from build123d import *

# Parameters (mm, degrees)
F1_DEPTH = 12.7
F2_SIZE  = 1.5875
F3_R     = 3.175
F8_ANGLE = 90


with BuildPart() as f1:
    # F0 (on Top) → F1 (new body)
    with BuildSketch(Plane.XY):
        with BuildLine():
            Line((25.4, 20.6375), (-12.7, 20.6375))
            ThreePointArc((-12.7, 20.6375), (-21.6802561211, 16.9177561211), (-25.4, 7.9375))
            Line((-25.4, 7.9375), (-25.4, -20.6375))
            Line((-25.4, -20.6375), (25.4, -20.6375))
            Line((25.4, -20.6375), (25.4, -5.55625))
            Line((25.4, -5.55625), (22.1241805311, -5.55625))
            ThreePointArc((22.1241805311, -5.55625), (21.2950640303, -7.0075640303), (19.84375, -7.8366805311))
            Line((19.84375, -7.8366805311), (19.84375, -11.2133194689))
            ThreePointArc((19.84375, -11.2133194689), (21.5600578928, -12.3432175167), (22.225, -14.2875))
            ThreePointArc((22.225, -14.2875), (17.1057175167, -16.7975578928), (18.25625, -11.2133194689))
            Line((18.25625, -11.2133194689), (18.25625, -7.8366805311))
            ThreePointArc((18.25625, -7.8366805311), (15.875, -4.7625), (18.25625, -1.6883194689))
            Line((18.25625, -1.6883194689), (18.25625, 1.6883194689))
            ThreePointArc((18.25625, 1.6883194689), (15.875, 4.7625), (18.25625, 7.8366805311))
            Line((18.25625, 7.8366805311), (18.25625, 11.2133194689))
            ThreePointArc((18.25625, 11.2133194689), (17.1057175167, 16.7975578928), (22.225, 14.2875))
            ThreePointArc((22.225, 14.2875), (21.5600578928, 12.3432175167), (19.84375, 11.2133194689))
            Line((19.84375, 11.2133194689), (19.84375, 7.8366805311))
            ThreePointArc((19.84375, 7.8366805311), (21.5600578928, 6.7067824833), (22.225, 4.7625))
            ThreePointArc((22.225, 4.7625), (21.5600578928, 2.8182175167), (19.84375, 1.6883194689))
            Line((19.84375, 1.6883194689), (19.84375, -1.6883194689))
            ThreePointArc((19.84375, -1.6883194689), (21.2950640303, -2.5174359697), (22.1241805311, -3.96875))
            Line((22.1241805311, -3.96875), (25.4, -3.96875))
            Line((25.4, -3.96875), (25.4, 20.6375))
        make_face()
        Polygon((-5.3676515813, 7.9375), (-9.0338257906, 1.5875), (-16.3661742094, 1.5875), (-20.0323484187, 7.9375), (-16.3661742094, 14.2875), (-9.0338257906, 14.2875), align=None, mode=Mode.SUBTRACT)
        with BuildLine():
            Line((19.84375, -11.2133194689), (19.84375, -7.8366805311))
            ThreePointArc((19.84375, -7.8366805311), (19.05, -7.9375), (18.25625, -7.8366805311))
            Line((18.25625, -7.8366805311), (18.25625, -11.2133194689))
            ThreePointArc((18.25625, -11.2133194689), (19.05, -11.1125), (19.84375, -11.2133194689))
        make_face()
        with BuildLine():
            ThreePointArc((18.25625, -1.6883194689), (19.05, -1.5875), (19.84375, -1.6883194689))
            Line((19.84375, -1.6883194689), (19.84375, 1.6883194689))
            ThreePointArc((19.84375, 1.6883194689), (19.05, 1.5875), (18.25625, 1.6883194689))
            Line((18.25625, 1.6883194689), (18.25625, -1.6883194689))
        make_face()
    extrude(amount=F1_DEPTH)

    # F2
    f2_edges = [f1.edges().sort_by_distance(p)[0] for p in [
        (19.05, 1.5875, 12.7),
        (19.05, 17.4625, 12.7),
        (18.25625, 9.525, 12.7),
        (19.84375, 9.525, 12.7),
    ]]
    chamfer(f2_edges, length=F2_SIZE)

    # F3
    f3_edges = [f1.edges().sort_by_distance(p)[0] for p in [
        (-7.200739, 4.7625, 12.7),
        (-7.200739, 11.1125, 12.7),
        (-12.7, 14.2875, 12.7),
        (-18.199261, 11.1125, 12.7),
        (-18.199261, 4.7625, 12.7),
        (-12.7, 1.5875, 12.7),
        (-16.366174, 14.2875, 6.35),
        (-20.032348, 7.9375, 6.35),
        (-16.366174, 1.5875, 6.35),
        (-9.033826, 1.5875, 6.35),
        (-5.367652, 7.9375, 6.35),
        (-9.033826, 14.2875, 6.35),
    ]]
    fillet(f3_edges, radius=F3_R)

    # F5 (on face) → F6 section 0
    with BuildSketch(Plane(origin=(0, 0, 0), x_dir=(1, 0, 0), z_dir=(0, 0, -1))):
        Polygon((-6.35, 11.0185455743), (-6.35, 3.6861971556), (0, 0.0200229463), (6.35, 3.6861971556), (6.35, 11.0185455743), (0, 14.6847197837), align=None)
    # F4 (on face) → F6 section 1
    with BuildSketch(Plane.XY.offset(12.7)):
        Polygon((2.749630657, -2.589871365), (-2.749630657, -2.589871365), (-5.499261314, -7.352371365), (-2.749630657, -12.114871365), (2.749630657, -12.114871365), (5.499261314, -7.352371365), align=None)
    loft(mode=Mode.SUBTRACT)

    # F7 (on face) → F8 (revolve)
    with BuildSketch(Plane.XZ.offset(20.6375)):
        with BuildLine():
            Line((-25.4, 12.7), (-6.35, 12.7))
            ThreePointArc((-6.35, 12.7), (-15.875, 22.225), (-25.4, 12.7))
        make_face()
    revolve(axis=Axis((-15.875, -20.6375, 12.7), (-1, 0, 0)), revolution_arc=F8_ANGLE)


solid = f1.part
Can you work these out from the model? Positions are in its coordinate system, mm. A direction names the side the tool comes from. Give positions to 0.01 mm unless a question says otherwise; leave off trailing zeros. Loops run counter-clockwise (first coordinate to the right, second up) from the corner with the lowest first, then second, coordinate; pieces in that order, holes last. Notation, with made-up numbers: (59, -31.75) - (81, -31.75) arc R32 cw to (81, 5.25) - close; hole circle Ø7 at (58, 32). An arc over 180 degrees is marked (long way). Return JSON: item names as keys, results as strings.
1. I'm going to push flat-ended pins straight in: pin 1 Ø1.7 at (y, z) = (10, 5) entering from -X; pin 2 Ø2 at (x, y) = (-19.5, -16) entering from +Z; pin 3 Ø20.5 at (x, y) = (1, -5) entering from +Z. Where does each tip first touch, or does it pass through?
Output values:
{"pin 1": "stops at x = -25.34", "pin 2": "stops at z = 20.88", "pin 3": "stops at z = 12.7"}
2. I want a section at A-A on x = 19.05. Please give me the cut outline in (y, z), and give its area (3 significant figures).
Output values:
{"outline": "(-20.64, 0) - (-17.46, 0) - (-17.46, 12.7) - (-20.64, 12.7) - close; (-11.11, 0) - (-7.94, 0) - (-7.94, 12.7) - (-11.11, 12.7) - close; (-1.59, 0) - (1.59, 0) - (1.59, 11.11) - (0, 12.7) - (-1.59, 12.7) - close; (17.46, 0) - (20.64, 0) - (20.64, 12.7) - (19.05, 12.7) - (17.46, 11.11) - close", "area": "159 mm²"}
3. We'd pull the mould along Y, two halves only. Please class faces 1 (the face through (-6, -20.638, 9)), 2 (the face through (-5.86, 7.96, 4.83)), 3 (the face through (25.4, -13, 6)): +Y half, -Y half, draft (parallel to the pull), parting line (faces both ways), or undercut.
Output values:
{"face 1": "-Y half", "face 2": "undercut", "face 3": "draft"}
4. If I drill on line 1 (Y direction, x = 19.05, z = 8.25); line 2 (Y direction, x = -12, z = 6.5); line 3 (Z direction, x = 17, y = 0), over which ranges is the centre line in solid material (lowest first)?
Output values:
{"line 1": "y = -20.64 to -17.46, -11.11 to -7.94, -1.59 to 1.59, 17.46 to 20.64", "line 2": "y = -20.64 to 1.59, 14.29 to 20.64", "line 3": "z = 0 to 12.7"}
5. I want a section at C-C on z = 1.5. Give the number of separate pieces and of enclosed holes in the cut face, and give its area (3 significant figures).
Output values:
{"separate pieces": "1", "enclosed holes": "4", "area": "1,660 mm²"}
6. For faces 4 (the face through (24, -3.969, 6)), 5 (the face through (-19.039, 4.307, 11.795)), 6 (the face through (-9.3, 2, 4.8)), which set-ups out of +Z, -Z, +X, -X, +Y, -Y let a thin tool reach every point of the face, with its end or its side?
Output values:
{"face 4": "+Z, -Z, +X", "face 5": "+Z", "face 6": "+Z, -Z"}
